Geometry: final body of the model. Coordinates: model frame, mm. Face numbers are marked on the shaded views. A direction names the side the tool comes from. Give positions to 0.01 mm unless a question says otherwise; leave off trailing zeros. Loops run counter-clockwise (first coordinate to the right, second up) from the corner with the lowest first, then second, coordinate; pieces in that order, holes last. Notation, with made-up numbers: (71.5, 22.25) - (108.5, 22.25) arc R27 ccw to (108.5, 45.25) - close; hole circle Ø5 at (52.5, 89). An arc over 180 degrees is marked (long way). Use one line per item in the form item = value.
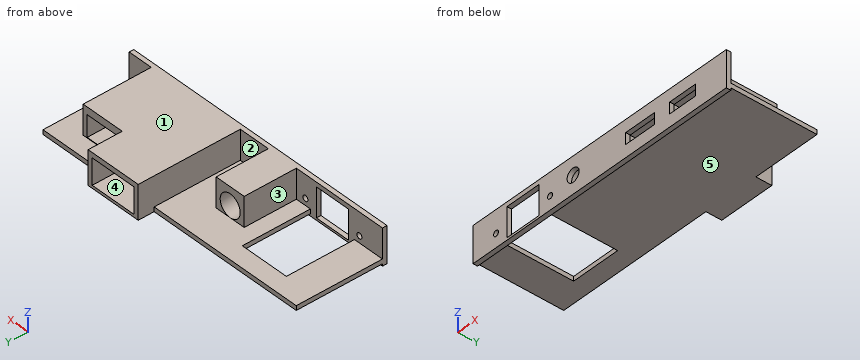
```python
from build123d import *

# Parameters (mm, degrees)
SKETCH_W        = 126.5
SKETCH_H        = 40
PAD_DEPTH       = 3
SKETCH001_W     = 126.5
SKETCH001_H     = 38
POCKET_DEPTH    = 1
SKETCH002_W     = 126.5
SKETCH002_H     = 2
PAD001_DEPTH    = 13
SKETCH003_W     = 19.5
SKETCH003_H     = 30
SKETCH003_W_2   = 25
SKETCH003_H_2   = 45
PAD002_DEPTH    = 15
SKETCH004_W     = 13
SKETCH004_H     = 5
POCKET001_DEPTH = 32.001
SKETCH005_W     = 17.5
SKETCH005_H     = 9.5
POCKET002_DEPTH = 30
SKETCH006_W     = 14.5
SKETCH006_H     = 5
POCKET003_DEPTH = 47.001
SKETCH007_W     = 21
SKETCH007_H     = 11.5
POCKET004_DEPTH = 45
SKETCH008_W     = 14
SKETCH008_H     = 23
PAD003_DEPTH    = 13
SKETCH009_R     = 5
POCKET005_DEPTH = 23
SKETCH010_R     = 3
POCKET006_DEPTH = 2.001
SKETCH011_R     = 1.25
SKETCH011_W     = 16
SKETCH011_H     = 13
POCKET007_DEPTH = 2
SKETCH012_W     = 22
SKETCH012_H     = 30
POCKET008_DEPTH = 3.001


with BuildPart() as part:
    # Sketch → Pad (new body)
    with BuildSketch(Plane.XY):
        with Locations((0, 20)):
            Rectangle(SKETCH_W, SKETCH_H)
    extrude(amount=PAD_DEPTH)

    # Sketch001 → Pocket (cut)
    with BuildSketch(Plane(origin=(0, 0, 0), x_dir=(1, 0, 0), z_dir=(0, 0, -1))):
        with Locations((0, -21)):
            Rectangle(SKETCH001_W, SKETCH001_H)
    extrude(amount=-POCKET_DEPTH, mode=Mode.SUBTRACT)

    # Sketch002 → Pad001 (new body)
    with BuildSketch(Plane.XY.offset(3)):
        with Locations((0, 1)):
            Rectangle(SKETCH002_W, SKETCH002_H)
    extrude(amount=PAD001_DEPTH)

    # Sketch003 → Pad002 (new body)
    with BuildSketch(Plane(origin=(0, 0, 1), x_dir=(1, 0, 0), z_dir=(0, 0, -1))):
        with Locations((42.5, -17)):
            Rectangle(SKETCH003_W, SKETCH003_H)
        with Locations((20.25, -24.5)):
            Rectangle(SKETCH003_W_2, SKETCH003_H_2)
    extrude(amount=-PAD002_DEPTH)

    # Sketch004 → Pocket001 (cut, through all)
    with BuildSketch(Plane(origin=(0, 32, 0), x_dir=(-1, 0, 0), z_dir=(0, 1, 0))):
        with Locations((-41.5, 8)):
            Rectangle(SKETCH004_W, SKETCH004_H)
    extrude(amount=-POCKET001_DEPTH, mode=Mode.SUBTRACT)

    # Sketch005 → Pocket002 (cut)
    with BuildSketch(Plane(origin=(0, 32, 0), x_dir=(-1, 0, 0), z_dir=(0, 1, 0))):
        with Locations((-41.5, 8)):
            Rectangle(SKETCH005_W, SKETCH005_H)
    extrude(amount=-POCKET002_DEPTH, mode=Mode.SUBTRACT)

    # Sketch006 → Pocket003 (cut, through all)
    with BuildSketch(Plane(origin=(0, 47, 0), x_dir=(-1, 0, 0), z_dir=(0, 1, 0))):
        with Locations((-20.25, 8)):
            Rectangle(SKETCH006_W, SKETCH006_H)
    extrude(amount=-POCKET003_DEPTH, mode=Mode.SUBTRACT)

    # Sketch007 → Pocket004 (cut)
    with BuildSketch(Plane(origin=(0, 47, 0), x_dir=(-1, 0, 0), z_dir=(0, 1, 0))):
        with Locations((-20.25, 8)):
            Rectangle(SKETCH007_W, SKETCH007_H)
    extrude(amount=-POCKET004_DEPTH, mode=Mode.SUBTRACT)

    # Sketch008 → Pad003 (new body)
    with BuildSketch(Plane.XY.offset(3)):
        with Locations((-13.25, 13.5)):
            Rectangle(SKETCH008_W, SKETCH008_H)
    extrude(amount=PAD003_DEPTH)

    # Sketch009 → Pocket005 (cut)
    with BuildSketch(Plane(origin=(0, 25, 0), x_dir=(-1, 0, 0), z_dir=(0, 1, 0))):
        with Locations((13.25, 8)):
            Circle(SKETCH009_R)
    extrude(amount=-POCKET005_DEPTH, mode=Mode.SUBTRACT)

    # Sketch010 → Pocket006 (cut, through all)
    with BuildSketch(Plane(origin=(0, 2, 0), x_dir=(-1, 0, 0), z_dir=(0, 1, 0))):
        with Locations((13.25, 8)):
            Circle(SKETCH010_R)
    extrude(amount=-POCKET006_DEPTH, mode=Mode.SUBTRACT)

    # Sketch011 → Pocket007 (cut)
    with BuildSketch(Plane.XZ):
        with Locations((-24.75, 6)):
            Circle(SKETCH011_R)
        with Locations((-51.75, 6)):
            Circle(SKETCH011_R)
        with Locations((-38.25, 7.5)):
            Rectangle(SKETCH011_W, SKETCH011_H)
    extrude(amount=-POCKET007_DEPTH, mode=Mode.SUBTRACT)

    # Sketch012 → Pocket008 (cut, through all)
    with BuildSketch(Plane.XY.offset(3)):
        with Locations((-38.25, 17)):
            Rectangle(SKETCH012_W, SKETCH012_H)
    extrude(amount=-POCKET008_DEPTH, mode=Mode.SUBTRACT)


solid = part.part
```
(1) Material intervals for L1, parallel to X at y = 18.5, z = 8; L2, parallel to Z at x = -51.75, y = 1.2; L3, parallel to Z at x = -13.25, y = 7, sorted ascending. Write a range as from..to.
Solution:
L1 = -20.25..-18.25, -8.25..-6.25, 7.75..9.75, 30.75..32.75, 50.25..52.25
L2 = 0..4.75, 7.25..16
L3 = 1..3, 13..16
(2) Pin query (flat end, axial travel): P1, Ø6, axis at y = 8.5, z = 8.5, coming from the -X side; P2, Ø4, axis at y = 15.5, z = 7, coming from the +X side; P3, Ø8, axis at x = 42.5, y = 34, coming from the -Z side. Return the tip coordinate at first contact, or that it passes through.
Solution:
P1 = -20.25
P2 = 52.25
P3 = 1
(3) Cut plane A-A (y = 9). Return the cut outline in (x, z).
Solution:
outline = (-63.25, 1) - (-49.25, 1) - (-49.25, 3) - (-63.25, 3) - close; (-27.25, 1) - (63.25, 1) - (63.25, 3) - (52.25, 3) - (52.25, 16) - (7.75, 16) - (7.75, 3) - (-6.25, 3) - (-6.25, 16) - (-20.25, 16) - (-20.25, 3) - (-27.25, 3) - close; hole circle Ø10 at (-13.25, 8); hole (9.75, 2.25) - (30.75, 2.25) - (30.75, 13.75) - (9.75, 13.75) - close; hole (32.75, 3.25) - (50.25, 3.25) - (50.25, 12.75) - (32.75, 12.75) - close
(4) Pull-direction query (X, two-part tool) for the marked faces 3, 4 and 5; classes: released by +X, released by -X, zero draft, split by the parting line, or undercut.
Solution:
face_3 = released by -X
face_4 = undercut
face_5 = zero draft
(5) Access query for the marked faces 1 and 2. Directions: +Z, -Z, +X, -X, +Y, -Y. A direction counts if a zero-diameter tool reaches every point of the face in a straight line with its end or side. Return the directions, or none.
Solution:
face_1 = +Z, +X, -X, +Y, -Y
face_2 = +Z, +Y
(6) Cut plane D-D (x = -4). Return the cut outline in (y, z).
Solution:
outline = (0, 0) - (2, 0) - (2, 1) - (40, 1) - (40, 3) - (2, 3) - (2, 16) - (0, 16) - close
(7) Cut plane C-C (x = 20.5). Return the cut outline in (y, z).
Solution:
outline = (0, 0) - (2, 0) - (2, 1) - (47, 1) - (47, 2.25) - (2, 2.25) - (2, 5.5) - (0, 5.5) - close; (0, 10.5) - (2, 10.5) - (2, 13.75) - (47, 13.75) - (47, 16) - (0, 16) - close
(8) Cut plane B-B (y = 27.5). Return the cut outline in (x, z).
Solution:
outline = (-63.25, 1) - (-49.25, 1) - (-49.25, 3) - (-63.25, 3) - close; (-27.25, 1) - (63.25, 1) - (63.25, 3) - (52.25, 3) - (52.25, 16) - (7.75, 16) - (7.75, 3) - (-27.25, 3) - close; hole (9.75, 2.25) - (30.75, 2.25) - (30.75, 13.75) - (9.75, 13.75) - close; hole (32.75, 3.25) - (50.25, 3.25) - (50.25, 12.75) - (32.75, 12.75) - close
